from build123d import *

# Parameters (mm, degrees)
CROQUIS1_R              = 11
SALIENTE_EXTRUIR1_DEPTH = 12
CROQUIS3_R              = 16
CORTAR_EXTRUIR2_DEPTH   = 10


with BuildPart() as part:
    # Croquis1 → Saliente-Extruir1 (new body)
    with BuildSketch(Plane.XY):
        with BuildLine():
            ThreePointArc((-26.771248385, 16.522500226), (-57.87296723, 15.696010738), (-57.046477743, -15.405708107))
            ThreePointArc((-57.046477743, -15.405708107), (-4.408863064, -36.394164074), (48.228751615, -15.405708107))
            ThreePointArc((48.228751615, -15.405708107), (49.055241102, 15.696010738), (17.953522257, 16.522500226))
            ThreePointArc((17.953522257, 16.522500226), (-4.408863064, 7.605835926), (-26.771248385, 16.522500226))
        make_face()
        with Locations((-41.908863064, 0.558396059)):
            Circle(CROQUIS1_R, mode=Mode.SUBTRACT)
        with Locations((33.091136936, 0.558396059)):
            Circle(CROQUIS1_R, mode=Mode.SUBTRACT)
    extrude(amount=SALIENTE_EXTRUIR1_DEPTH)

    # Croquis3 → Cortar-Extruir2 (cut)
    with BuildSketch(Plane(origin=(0, 0, 0), x_dir=(-1, 0, 0), z_dir=(0, 0, -1))):
        with Locations((41.908863064, 0.558396059)):
            Circle(CROQUIS3_R)
        with Locations((-33.091136936, 0.558396059)):
            Circle(CROQUIS3_R)
    extrude(amount=-CORTAR_EXTRUIR2_DEPTH, mode=Mode.SUBTRACT)


solid = part.part
Can you work these out from the model? Positions are in its coordinate system, mm. A direction names the side the tool comes from. Coordinates: 2 decimals unless noted, no trailing zeros. Write each loop counter-clockwise with the first axis right and the second up, starting at its lowest first coordinate (ties: lowest second). Pieces come first, ordered by that corner, then holes.
Q1. Imagine slicing it at D-D, the plane x = 46. List the corners of the cut face in (y, z) for me, plus the area to 3 significant figures.
Results found:
outline: (-17.44, 0) - (-8.89, 0) - (-8.89, 10) - (10.01, 10) - (10.01, 0) - (18.37, 0) - (18.37, 12) - (-17.44, 12) - close
area: 241 mm2
Q2. Which directions (+Z, -Z, +X, -X, +Y, -Y) give clear straight access to the entire face, cutting with the end or side of a thin tool? Please do faces 4 (the face through (37, -10, 10)), 5 (the face through (-5, -7, 12)).
Results found:
face 4: -Z
face 5: +Z, +X, -X, +Y, -Y
Q3. Please list where these lines run through material, in increasing order: L1, parallel to X at y = 0, z = 2; L2, parallel to X at y = -9.5, z = 5.25; L3, parallel to X at y = 18.5, z = 1.5.
Results found:
L1: x = -63.9 to -57.9, -25.92 to 17.1, 49.08 to 55.08
L2: x = -61.47 to -54.35, -29.47 to 20.65, 45.53 to 52.66
L3: x = -54.64 to -29.18, 20.36 to 45.82
Q4. For P1, Ø19, axis at x = -41.91, y = 0.56, coming from the +Z side; P2, Ø16, axis at x = -47.5, y = 3.5, coming from the -Z side; P3, Ø3, axis at y = -7, z = 6.5, coming from the +X side; P4, Ø3, axis at x = -18, z = 10, coming from the -Y side, each with a flat end and sliding along its axis, tell me the tip position at first contact or that it passes through.
Results found:
P1: passes through
P2: stops at z = 10
P3: stops at x = 54.24
P4: stops at y = -35.43
Q5. Imagine slicing it at B-B, the plane y = -6.5. List the corners of the cut face in (x, z) for me.
Results found:
outline: (-62.75, 0) - (-56.27, 0) - (-56.27, 10) - (-50.35, 10) - (-50.35, 12) - (-62.75, 12) - close; (-33.47, 10) - (-27.55, 10) - (-27.55, 0) - (18.73, 0) - (18.73, 10) - (24.65, 10) - (24.65, 12) - (-33.47, 12) - close; (41.53, 10) - (47.45, 10) - (47.45, 0) - (53.93, 0) - (53.93, 12) - (41.53, 12) - close
Q6. Imagine slicing it at A-A, the plane x = 27. List the corners of the cut face in (y, z) for me, plus the area to 3 significant figures.
Results found:
outline: (-29.65, 0) - (-14.24, 0) - (-14.24, 10) - (-8.6, 10) - (-8.6, 12) - (-29.65, 12) - close; (9.72, 10) - (15.35, 10) - (15.35, 0) - (21.7, 0) - (21.7, 12) - (9.72, 12) - close
area: 284 mm2
Q7. Imagine slicing it at C-C, the plane z = 5.5. List the corners of the cut face in (x, y) for me.
Results found:
outline: (-57.05, -15.41) arc R76.5 ccw to (48.23, -15.41) arc R22 ccw to (17.95, 16.52) arc R32.5 cw to (-26.77, 16.52) arc R22 ccw to start; hole circle Ø32 at (-41.91, 0.56); hole circle Ø32 at (33.09, 0.56)
Q8. If we mould it in two halves opening along Y, with no side actions, what happens to faces 1 (the face through (-57.17, 5.36, 4.93)), 2 (the face through (-4.064, 7.608, 5.916)), 3 (the face through (49.384, 15.341, 5.916))? For each: +Y half, -Y half, draft (parallel to the pull), parting line (faces both ways), or undercut.
Results found:
face 1: undercut
face 2: +Y half
face 3: parting line
